Here's how the part is built. I have some questions about the finished solid (model axes, mm). A direction names the side the tool comes from. Round coordinates to 2 decimals unless told otherwise and drop trailing zeros. Write each loop counter-clockwise with the first axis right and the second up, starting at its lowest first coordinate (ties: lowest second). Pieces come first, ordered by that corner, then holes. Notation, with made-up numbers: (74.5, -7) - (126.5, -7) arc R33 cw to (126.5, 32) - close; hole circle Ø2 at (-5.5, 33.5). An arc over 180 degrees is marked (long way). One line per question, with ' | ' between items. Start each with the question number.
(1) Thinking about a two-plate mould opening in Z: for faces 1 (the cylindrical face through (2, -0.1, -2.5)), 2 (the cylindrical face through (0.99, 3.955, -5.158)), 3 (the flat face through (2, 4, -3)), which applies, pulls with the +Z half, pulls with the -Z half, needs draft (parallel to the pull), parting line crosses it, or undercut?
(2) Imagine slicing it at A-A (y = 0). Write out the boundary of the cut face in (x, z).
(3) Will these pins go through, and if not, where does the flat tip stop? pin 1 (6 mm diameter, centred on y = -4, z = 2, fed in from +X); pin 2 (1 mm diameter, centred on x = 3.5, z = 2, fed in from -Y); pin 3 (2 mm diameter, centred on x = 2, y = -5, fed in from -Z); pin 4 (1.5 mm diameter, centred on x = 2, z = -1, fed in from +Y).
(4) If I drill on L1, parallel to Y at x = 1.4, z = 0; L2, parallel to Y at x = 3.3, z = 0.25; L3, parallel to X at y = -1, z = 4.75, over which ranges is the centre line in solid material (lowest first)?
(5) Imagine slicing it at C-C (x = 0.8). Write out the boundary of the cut face in (y, z).
(6) For faces 4 (the flat face through (4, 1, -3)), 5 (the cylindrical face through (2.99, -3.04, -3.32)), which set-ups out of +Z, -Z, +X, -X, +Y, -Y let a thin tool reach every point of the face, with its end or its side?
from build123d import *

# Parameters (mm, degrees)
ZAOBLIT1_R   = 0.3
ZKOSIT1_SIZE = 0.3


with BuildPart() as part:
    # Skica1 → Otočit kolem osy1 (revolve)
    with BuildSketch(Plane.XY, mode=Mode.PRIVATE) as oto_it_kolem_osy1_sk:
        Polygon((0, 2.5), (4, 2.5), (4, 4.5), (2, 4.5), (2, 6.5), (0, 6.5), align=None)
    revolve(oto_it_kolem_osy1_sk.sketch.rotate(Axis((0, 0, 0), (1, 0, 0)), 90), axis=Axis((0, 0, 0), (1, 0, 0)))

    # Zaoblit1
    zaoblit1_edges = [part.edges().sort_by_distance(p)[0] for p in [
        (2, 0, -4.5),
    ]]
    fillet(zaoblit1_edges, radius=ZAOBLIT1_R)

    # Zkosit1
    zkosit1_edges = [part.edges().sort_by_distance(p)[0] for p in [
        (0, 0, -6.5),
        (2, 0, -6.5),
        (4, 0, -4.5),
        (4, 0, -2.5),
        (0, 0, -2.5),
    ]]
    chamfer(zkosit1_edges, length=ZKOSIT1_SIZE)


solid = part.part
Check sheet entries:
1) face 1: undercut | face 2: parting line crosses it | face 3: needs draft
2) outline: (0, -6.2) - (0.3, -6.5) - (1.7, -6.5) - (2, -6.2) - (2, -4.8) arc R0.3 cw to (2.3, -4.5) - (3.7, -4.5) - (4, -4.2) - (4, -2.8) - (3.7, -2.5) - (0.3, -2.5) - (0, -2.8) - close; (0, 2.8) - (0.3, 2.5) - (3.7, 2.5) - (4, 2.8) - (4, 4.2) - (3.7, 4.5) - (2.3, 4.5) arc R0.3 cw to (2, 4.8) - (2, 6.2) - (1.7, 6.5) - (0.3, 6.5) - (0, 6.2) - close
3) pin 1: x = 4 | pin 2: y = -4.24 | pin 3: z = -5.09 | pin 4: y = 6.49
4) L1: -6.5 to -2.5, 2.5 to 6.5 | L2: -4.49 to -2.49, 2.49 to 4.49 | L3: 0 to 2
5) outline: circle Ø13 at (0, 0); hole circle Ø5 at (0, 0)
6) face 4: +Z, -Z, +X, +Y, -Y | face 5: +X
